```python
from build123d import *

# Parameters (mm, degrees)
SKETCH_1_W                  = 86
SKETCH_1_H                  = 86
EXTRUDE_1_DEPTH             = 6
SKETCH_2_W                  = 30
SKETCH_2_H                  = 30
EXTRUDE_2_DEPTH             = 160
EXTRUDE_3_REACH             = 173.167
EXTRUDE_3_DIRECTION_2_REACH = 173.167
SKETCH_8_R                  = 2.6
CUT_EXTRUDE_2_DEPTH         = 6
CUT_EXTRUDE_3_DEPTH         = 6
PATTERN_LINEAR_1_COUNT      = 2
PATTERN_LINEAR_1_PITCH      = 91.2
MIRROR_7_COPY_1_DEPTH       = 6
MIRROR_8_COPY_1_SKETCH_R    = 2.6
MIRROR_8_COPY_1_DEPTH       = 6
PATTERN_CIRCULAR_1_COUNT    = 2
PATTERN_CIRCULAR_1_ANGLE    = 90
MIRROR_9_COPY_1_SKETCH_R    = 2.6
MIRROR_9_COPY_1_DEPTH       = 6
MIRROR_9_COPY_2_SKETCH_R    = 2.6
MIRROR_9_COPY_2_DEPTH       = 6
MIRROR_10_COPY_1_SKETCH_R   = 2.6
MIRROR_10_COPY_1_DEPTH      = 6
MIRROR_10_COPY_2_SKETCH_R   = 2.6
MIRROR_10_COPY_2_DEPTH      = 6
MIRROR_10_COPY_3_SKETCH_R   = 2.6
MIRROR_10_COPY_3_DEPTH      = 6
MIRROR_10_COPY_4_SKETCH_R   = 2.6
MIRROR_10_COPY_4_DEPTH      = 6
MIRROR_10_COPY_5_SKETCH_R   = 2.6
MIRROR_10_COPY_5_DEPTH      = 6
EXTRUDE_4_DEPTH             = 15
CUT_EXTRUDE_START           = -172.166585524
SKETCH_17_W                 = 15.666596152
SKETCH_17_H                 = 20.507289597
CUT_EXTRUDE_4_DEPTH         = 177.166585524
SKETCH_18_R                 = 7.890659629
SKETCH_18_R_2               = 8.087611604
CUT_EXTRUDE_5_DEPTH         = 177.166585524
PATTERN_START               = -8.175929672
PATTERN_LINEAR_2_OUTLINE_W  = 20
PATTERN_LINEAR_2_OUTLINE_H  = 20.507289597
PATTERN_LINEAR_2_DEPTH      = 15.666596152
PATTERN_LINEAR_3_COUNT      = 3
PATTERN_LINEAR_3_PITCH      = 60


# Read off the part's stored shape, not the designer's step: 阵列(线性)2
with BuildPart() as part:
    # 草图1 → 凸台-拉伸1 (new body)
    with BuildSketch(Plane(origin=(0, 0, 0), x_dir=(1, 0, 0), z_dir=(0, 1, 0))):
        Rectangle(SKETCH_1_W, SKETCH_1_H)
    extrude(amount=EXTRUDE_1_DEPTH)

    # 草图2 → 凸台-拉伸2 (add)
    with BuildSketch(Plane(origin=(0, 0, 0), x_dir=(1, 0, 0), z_dir=(0, 1, 0))):
        Rectangle(SKETCH_2_W, SKETCH_2_H)
    extrude(amount=EXTRUDE_2_DEPTH)

    # 凸台-拉伸3: up to this face of the body (flat: up to its plane)
    extrude_3_end = Plane(part.part.faces().sort_by_distance((0, 83, 15))[0])
    # 草图7 → 凸台-拉伸3 (add, up to the picked face)
    with BuildSketch(Plane.XY, mode=Mode.PRIVATE) as extrude_3_sk1:
        Polygon((-15, 36), (-33, 6), (-15, 6), align=None)
    extrude_3_tool1 = split(extrude(extrude_3_sk1.sketch, amount=EXTRUDE_3_REACH, mode=Mode.PRIVATE), bisect_by=extrude_3_end, keep=Keep.BOTH, mode=Mode.PRIVATE)
    add(extrude_3_tool1.solids().sort_by(Axis((-21, 16, 0), (0, 0, 1)))[0])

    # 凸台-拉伸3 direction 2: up to this face of the body (flat: up to its plane)
    extrude_3_direction_2_end = Plane(part.part.faces().sort_by_distance((0, 83, -15))[0])
    # 草图7 → 凸台-拉伸3 direction 2 (add, up to the picked face)
    with BuildSketch(Plane.XY, mode=Mode.PRIVATE) as extrude_3_direction_2_sk1:
        Polygon((-15, 36), (-33, 6), (-15, 6), align=None)
    extrude_3_direction_2_tool1 = split(extrude(extrude_3_direction_2_sk1.sketch, amount=-EXTRUDE_3_DIRECTION_2_REACH, mode=Mode.PRIVATE), bisect_by=extrude_3_direction_2_end, keep=Keep.BOTH, mode=Mode.PRIVATE)
    add(extrude_3_direction_2_tool1.solids().sort_by(Axis((-21, 16, 0), (0, 0, -1)))[0])

    # 草图8 → 切除-拉伸2 (cut)
    with BuildSketch(Plane(origin=(0, 0, 0), x_dir=(1, 0, 0), z_dir=(0, 1, 0))):
        with Locations(Location((-12.4, 37.4, 0), (0, 0, 270))):
            Circle(SKETCH_8_R)
    cut_extrude_2 = extrude(amount=CUT_EXTRUDE_2_DEPTH, mode=Mode.SUBTRACT)

    # 镜向2: 切除-拉伸2 across plane
    add(cut_extrude_2.mirror(Plane.XY), mode=Mode.SUBTRACT)

    # 草图11 → 切除-拉伸3 (cut)
    with BuildSketch(Plane(origin=(0, 0, 0), x_dir=(1, 0, 0), z_dir=(0, 1, 0))):
        Polygon((264.106039705, -18.2), (43, -18.2), (18.2, -18.2), (18.2, -43), (18.2, -264.106039705), (330.891160074, -576.797199779), (576.797199779, -330.891160074), align=None)
    cut_extrude_3 = extrude(amount=CUT_EXTRUDE_3_DEPTH, mode=Mode.SUBTRACT)

    # 草图12 → 切除-旋转2 (revolve, cut)
    with BuildSketch(Plane.XY):
        with BuildLine():
            Line((15, 58.5), (15, 45.5))
            ThreePointArc((15, 45.5), (8.5, 52), (15, 58.5))
        make_face()
    cut_revolve_2 = revolve(axis=Axis((15, 58.5, 0), (0, -1, 0)), mode=Mode.SUBTRACT)

    # 阵列(线性)1: 切除-旋转2 ×2
    with Locations(*[(0, i * PATTERN_LINEAR_1_PITCH, 0) for i in range(1, PATTERN_LINEAR_1_COUNT)]):
        add(cut_revolve_2, mode=Mode.SUBTRACT)

    # 镜向6: 切除-拉伸3 across plane
    add(cut_extrude_3.mirror(Plane.XY), mode=Mode.SUBTRACT)

    # 镜向7: 切除-拉伸3 across plane
    add(cut_extrude_3.mirror(Plane(origin=(0, 0, 0), x_dir=(0, 0, 1), z_dir=(1, 0, 0))), mode=Mode.SUBTRACT)

    # 镜向7 copy 1 sketch → 镜向7 copy 1 (cut)
    with BuildSketch(Plane(origin=(0, 0, 0), x_dir=(-1, 0, 0), z_dir=(0, 1, 0))):
        Polygon((264.106039705, -18.2), (43, -18.2), (18.2, -18.2), (18.2, -43), (18.2, -264.106039705), (330.891160074, -576.797199779), (576.797199779, -330.891160074), align=None)
    extrude(amount=MIRROR_7_COPY_1_DEPTH, mode=Mode.SUBTRACT)

    # 镜向8: 切除-拉伸2 across plane
    add(cut_extrude_2.mirror(Plane(origin=(0, 0, 0), x_dir=(0, 0, 1), z_dir=(1, 0, 0))), mode=Mode.SUBTRACT)

    # 镜向8 copy 1 sketch → 镜向8 copy 1 (cut)
    with BuildSketch(Plane(origin=(0, 0, 0), x_dir=(-1, 0, 0), z_dir=(0, 1, 0))):
        with Locations(Location((-12.4, 37.4, 0), (0, 0, 270))):
            Circle(MIRROR_8_COPY_1_SKETCH_R)
    extrude(amount=MIRROR_8_COPY_1_DEPTH, mode=Mode.SUBTRACT)

    # 阵列(圆周)1: 切除-拉伸2 ×2 about axis
    pattern_circular_1_axis = Axis((0, 0, 0), (0, 1, 0))
    for i in range(1, PATTERN_CIRCULAR_1_COUNT):
        add(cut_extrude_2.rotate(pattern_circular_1_axis, i * PATTERN_CIRCULAR_1_ANGLE / (PATTERN_CIRCULAR_1_COUNT - 1)), mode=Mode.SUBTRACT)

    # 镜向9 copy 1 sketch → 镜向9 copy 1 (cut)
    with BuildSketch(Plane.ZX):
        with Locations((-12.4, -37.4)):
            Circle(MIRROR_9_COPY_1_SKETCH_R)
    extrude(amount=MIRROR_9_COPY_1_DEPTH, mode=Mode.SUBTRACT)

    # 镜向9 copy 2 sketch → 镜向9 copy 2 (cut)
    with BuildSketch(Plane(origin=(0, 0, 0), x_dir=(1, 0, 0), z_dir=(0, 1, 0))):
        with Locations((-12.4, -37.4)):
            Circle(MIRROR_9_COPY_2_SKETCH_R)
    extrude(amount=MIRROR_9_COPY_2_DEPTH, mode=Mode.SUBTRACT)

    # 镜向10 copy 1 sketch → 镜向10 copy 1 (cut)
    with BuildSketch(Plane(origin=(0, 0, 0), x_dir=(0, 0, -1), z_dir=(0, 1, 0))):
        with Locations((-12.4, -37.4)):
            Circle(MIRROR_10_COPY_1_SKETCH_R)
    extrude(amount=MIRROR_10_COPY_1_DEPTH, mode=Mode.SUBTRACT)

    # 镜向10 copy 2 sketch → 镜向10 copy 2 (cut)
    with BuildSketch(Plane(origin=(0, 0, 0), x_dir=(-1, 0, 0), z_dir=(0, 1, 0))):
        with Locations((-12.4, -37.4)):
            Circle(MIRROR_10_COPY_2_SKETCH_R)
    extrude(amount=MIRROR_10_COPY_2_DEPTH, mode=Mode.SUBTRACT)

    # 镜向10 copy 3 sketch → 镜向10 copy 3 (cut)
    with BuildSketch(Plane.ZX):
        with Locations(Location((-12.4, 37.4, 0), (0, 0, 270))):
            Circle(MIRROR_10_COPY_3_SKETCH_R)
    extrude(amount=MIRROR_10_COPY_3_DEPTH, mode=Mode.SUBTRACT)

    # 镜向10 copy 4 sketch → 镜向10 copy 4 (cut)
    with BuildSketch(Plane(origin=(0, 0, 0), x_dir=(-1, 0, 0), z_dir=(0, 1, 0))):
        with Locations(Location((-12.4, 37.4, 0), (0, 0, 270))):
            Circle(MIRROR_10_COPY_4_SKETCH_R)
    extrude(amount=MIRROR_10_COPY_4_DEPTH, mode=Mode.SUBTRACT)

    # 镜向10 copy 5 sketch → 镜向10 copy 5 (cut)
    with BuildSketch(Plane(origin=(0, 0, 0), x_dir=(-1, 0, 0), z_dir=(0, 1, 0))):
        with Locations((-12.4, -37.4)):
            Circle(MIRROR_10_COPY_5_SKETCH_R)
    extrude(amount=MIRROR_10_COPY_5_DEPTH, mode=Mode.SUBTRACT)

    # 草图15 → 凸台-拉伸4 (add, symmetric)
    with BuildSketch(Plane(origin=(0, 0, 0), x_dir=(0, 0, -1), z_dir=(1, 0, 0))):
        Polygon((-15, 36), (-15, 6), (-33, 6), align=None)
    extrude_4 = extrude(amount=EXTRUDE_4_DEPTH, both=True)

    # 镜向11: 凸台-拉伸4 across plane
    add(extrude_4.mirror(Plane.XY))

    # 草图16 → 切除-旋转3 (revolve, cut)
    with BuildSketch(Plane.XY):
        with BuildLine():
            Line((15, 102.1), (15, 93.1))
            ThreePointArc((15, 93.1), (19.5, 97.6), (15, 102.1))
        make_face()
    revolve(axis=Axis((15, 102.1, 0), (0, -1, 0)), mode=Mode.SUBTRACT)

    # 草图17 → 切除-拉伸4 (cut)
    with BuildSketch(Plane(origin=(0, 0, 0), x_dir=(0, 0, -1), z_dir=(1, 0, 0)).offset(CUT_EXTRUDE_START)):
        with Locations((0.342631596, 141.05128602)):
            Rectangle(SKETCH_17_W, SKETCH_17_H)
    extrude(amount=CUT_EXTRUDE_4_DEPTH, mode=Mode.SUBTRACT)

    # 草图18 → 切除-拉伸5 (cut)
    with BuildSketch(Plane(origin=(0, 0, 0), x_dir=(0, 0, -1), z_dir=(1, 0, 0)).offset(CUT_EXTRUDE_START)):
        with Locations((0.342631596, 151.304930818)):
            Circle(SKETCH_18_R)
        with Locations((0.342631596, 130.797641221)):
            Circle(SKETCH_18_R_2)
    cut_extrude_5 = extrude(amount=CUT_EXTRUDE_5_DEPTH, mode=Mode.SUBTRACT)

    # 阵列(线性)2 outline → 阵列(线性)2 (cut)
    with BuildSketch(Plane.XY.offset(PATTERN_START)):
        with Locations((-5, 81.051286019)):
            Rectangle(PATTERN_LINEAR_2_OUTLINE_W, PATTERN_LINEAR_2_OUTLINE_H)
        Polygon((5, 10.797641221), (5, 31.304930818), (-17.817041509, 31.304930818), (-30.121415267, 10.797641221), align=None)
    extrude(amount=PATTERN_LINEAR_2_DEPTH, mode=Mode.SUBTRACT)

    # 阵列(线性)3: 切除-拉伸5 ×3
    with Locations(*[(0, -i * PATTERN_LINEAR_3_PITCH, 0) for i in range(1, PATTERN_LINEAR_3_COUNT)]):
        add(cut_extrude_5, mode=Mode.SUBTRACT)


solid = part.part
```
Geometry: final body of the model. Coordinates: model frame, mm. A direction names the side the tool comes from. Round coordinates to 2 decimals unless told otherwise and drop trailing zeros. Order: outer loops, then holes, each group sorted by start corner. A loop starts at its lowest first (then second) coordinate and runs counter-clockwise, first axis right, second up. Notation, with made-up numbers: (81, 72.25) -> (111, 72.25) arc R18 cw to (111, 94.25) -> close; hole circle Ø3 at (-18, 63). An arc over 180 degrees is marked (long way). Use CSV: the item, a comma, the result in double quotes. Start each with the question number.
1) Draft query along Y for faces 1 (the face through (18.2, 3, 30)), 2 (the face through (-19.336, 2.713, -0.136)), 3 (the face through (0, 160, 0)). Return one class per face: +Y half, -Y half, draft (parallel to the pull), parting line (faces both ways), or undercut.
2) Section A-A (x = -12.4). State how many separate pieces and enclosed holes the cut face has, and give its area (3 significant figures).
3) Section D-D (y = 26.5). Return the cut outline in (x, z).
4) Set-up query: faces 4 (the face through (-15, 15, -20)), 5 (the face through (31, 3, -18.2)), 6 (the face through (0, 99, 15)), 7 (the face through (-5.14, 122.713, -0.136)). Return all of +Z, -Z, +X, -X, +Y, -Y with unobstructed straight access to the full face (end or side cutting, diameter ignored); none if empty.
5) Section B-B (z = -12.4). Return the cut outline in (x, y).
6) Section C-C (x = 37.4). Return the cut outline in (y, z).
7) First-contact query: pin 1 Ø7 at (x, z) = (-37.4, 12.4) entering from +Y; pin 2 Ø14 at (y, z) = (151.3, -0.34) entering from +X; pin 3 Ø1.8 at (x, y) = (-25, 3) entering from -Z. Flat tips, straight axial feed; report the tip coordinate or a pass-through.
8) Material intervals for line 1 along X through (y, z) = (1, 37); line 2 along Z through (x, y) = (-3.5, 136); line 3 along Z through (x, y) = (-8.5, 112), sorted ascending. Write a range as from..to.
Returned:
1,face 1,"draft"
1,face 2,"undercut"
1,face 3,"+Y half"
2,separate pieces,"3"
2,enclosed holes,"3"
2,area,"4,050 mm²"
3,outline,"(-20.7, -15) -> (-15, -15) -> (-15, -20.7) -> (15, -20.7) -> (15, 20.7) -> (-15, 20.7) -> (-15, 15) -> (-20.7, 15) -> (-20.7, 7.49) -> (5, 7.49) -> (5, -8.18) -> (-20.7, -8.18) -> close"
4,face 4,"-Z, -X, +Y"
4,face 5,"-Z, +X, +Y, -Y"
4,face 6,"+Z, +X, -X, +Y"
4,face 7,"-X"
5,outline,"(-43, 0) -> (-40, 0) -> (-40, 6) -> (-43, 6) -> close; (-34.8, 0) -> (34.8, 0) -> (34.8, 6) -> (15, 6) -> (15, 160) -> (-15, 160) -> (-15, 36) -> (-33, 6) -> (-34.8, 6) -> close; (40, 0) -> (43, 0) -> (43, 6) -> (40, 6) -> close"
6,outline,"(0, -18.2) -> (6, -18.2) -> (6, -15) -> (0, -15) -> close; (0, -9.8) -> (6, -9.8) -> (6, 9.8) -> (0, 9.8) -> close; (0, 15) -> (6, 15) -> (6, 18.2) -> (0, 18.2) -> close"
7,pin 1,"stops at y = 6"
7,pin 2,"stops at x = 15"
7,pin 3,"stops at z = -18.2"
8,line 1,"x = -18.2..-14.97, -9.83..9.83, 14.97..18.2"
8,line 2,"z = -15..-8.18, 7.49..15"
8,line 3,"z = -15..15"
